Check sheet for the modelled part. Datum: model origin and axes. Units: mm. A direction names the side the tool comes from. Round coordinates to 2 decimals unless told otherwise and drop trailing zeros. Write each loop counter-clockwise with the first axis right and the second up, starting at its lowest first coordinate (ties: lowest second). Pieces come first, ordered by that corner, then holes. Notation, with made-up numbers: (82, 38) -> (109, 38) arc R16 ccw to (109, 68) -> close; hole circle Ø3 at (-4, -38.75). An arc over 180 degrees is marked (long way). Use one line per item in the form item = value. Start each with the question number.
```python
from build123d import *

# Parameters (mm, degrees)
SKETCH_2_R                   = 12
EXTRUDE_1_DEPTH              = 3.5
SKETCH_3_R                   = 2.95
EXTRUDE_2_DEPTH              = 2
HOLE_WIZARD_M3_1_D           = 3.4
HOLE_WIZARD_M3_1_CBORE_D     = 6.5
HOLE_WIZARD_M3_1_CBORE_DEPTH = 1.5
PATTERN_CIRCULAR_1_COUNT     = 4


with BuildPart() as part:
    # 草图1 → 旋转1 (revolve)
    with BuildSketch(Plane.XY, mode=Mode.PRIVATE) as revolve_1_sk:
        Polygon((3, 27.3), (3, 28.5), (0, 28.5), (0, 0), (3.5, 0), (3.5, 3.5), (3, 3.5), (3, 26.5), (2.6, 26.5), (2.6, 27.3), align=None)
    revolve(revolve_1_sk.sketch.rotate(Axis((0, 0, 0), (0, 1, 0)), 90), axis=Axis((0, 0, 0), (0, 1, 0)))

    # 草图2 → 凸台-拉伸1 (add)
    with BuildSketch(Plane.XZ):
        with Locations(Location((0, 0, 0), (0, 0, 270))):
            Circle(SKETCH_2_R)
    extrude(amount=EXTRUDE_1_DEPTH)

    # 草图3 → 凸台-拉伸2 (add)
    with BuildSketch(Plane.XZ.offset(3.5)):
        with Locations(Location((0, 0, 0), (0, 0, 270))):
            Circle(SKETCH_3_R)
    extrude(amount=EXTRUDE_2_DEPTH)

    # M3 六角凹头螺钉的柱形沉头孔1 (through all)
    with Locations(Plane(origin=(0, 0, 0), x_dir=(1, 0, 0), z_dir=(0, 1, 0))):
        with Locations((8.5, 0)):
            hole_wizard_m3_1 = CounterBoreHole(HOLE_WIZARD_M3_1_D / 2, HOLE_WIZARD_M3_1_CBORE_D / 2, HOLE_WIZARD_M3_1_CBORE_DEPTH)

    # 阵列(圆周)1: M3 六角凹头螺钉的柱形沉头孔1 ×4 about axis
    pattern_circular_1_axis = Axis((0, 0, 0), (0, 1, 0))
    for i in range(1, PATTERN_CIRCULAR_1_COUNT):
        add(hole_wizard_m3_1.rotate(pattern_circular_1_axis, i * 360 / PATTERN_CIRCULAR_1_COUNT), mode=Mode.SUBTRACT)


solid = part.part
```
1. Tool access check on faces 1 (the face through (-2.5, -3.5, -2.5)), 2 (the face through (0.07, -2.51, 10.2)), 3 (the face through (-0.9, 15.16, -2.86)). Record the directions out of +Z, -Z, +X, -X, +Y, -Y that give a thin tool (end or side, any length) a straight path to the whole face; none if there is none.
2. Sectioned sample at A-A (x = 0). Give the number of separate pieces and of enclosed holes in the cut face, and give its area (3 significant figures).
3. Mould release check, pull along X, two halves, no side actions. Record for faces 4 (the face through (0, 28.5, 0)), 5 (the face through (-1.4, -1.5, 9.9)), 6 (the face through (-2.88, -4.49, 0.64)), 7 (the face through (0.143, -0.74, 5.253)): +X half, -X half, draft (parallel to the pull), parting line (faces both ways), or undercut.
4. Sectioned sample at B-B (z = -8.5). Enter the section's corners in (x, y).
5. Depth check by flat-ended pin: pin 1 (3 mm diameter, centred on x = 0, z = -8.5, fed in from +Y); pin 2 (2 mm diameter, centred on x = -10, z = 0.5, fed in from +Y); pin 3 (7 mm diameter, centred on x = 0.5, z = 10, fed in from +Y); pin 4 (4 mm diameter, centred on x = -0.5, y = 15.5, fed in from -Z). Enter the tip coordinate at first touch or a pass-through.
6. Scan lines: probe 1 along Y at (x, z) = (-2.5, 1.5); probe 2 along Y at (x, z) = (1.25, -6); probe 3 along Y at (x, z) = (-6.5, 7.5). Record each from-to range of solid material in increasing order.
7. Sectioned sample at C-C (x = -9.75). Enter the section's corners in (y, z).
Returned:
q1.face_1 = -Y
q1.face_2 = +Y, -Y
q1.face_3 = +Y
q2.separate_pieces = 3
q2.enclosed_holes = 0
q2.area = 237 mm^2
q3.face_4 = draft
q3.face_5 = undercut
q3.face_6 = parting line
q3.face_7 = undercut
q4.outline = (-8.47, -3.5) -> (-1.7, -3.5) -> (-1.7, -1.5) -> (-3.25, -1.5) -> (-3.25, 0) -> (-8.47, 0) -> close; (1.7, -3.5) -> (8.47, -3.5) -> (8.47, 0) -> (3.25, 0) -> (3.25, -1.5) -> (1.7, -1.5) -> close
q5.pin_1 = through
q5.pin_2 = -1.5
q5.pin_3 = 0
q5.pin_4 = -3
q6.probe_1 = -5.5 to 26.5, 27.3 to 28.5
q6.probe_2 = -3.5 to -1.5
q6.probe_3 = -3.5 to 0
q7.outline = (-3.5, -7) -> (0, -7) -> (0, -3) -> (-1.5, -3) -> (-1.5, -1.15) -> (-3.5, -1.15) -> close; (-3.5, 1.15) -> (-1.5, 1.15) -> (-1.5, 3) -> (0, 3) -> (0, 7) -> (-3.5, 7) -> close
